Could you check a few things on this model? Use its own coordinates, in mm. Face numbers are marked on the shaded views. A direction names the side the tool comes from. Coordinates: 2 decimals unless noted, no trailing zeros. Loops run counter-clockwise (first coordinate to the right, second up) from the corner with the lowest first, then second, coordinate; pieces in that order, holes last.
Autodesk Inventor part; units mm, degrees
ref_plane "YZ Plane" through (0, 0, 0) normal (1, 0, 0) x (0, 1, 0)
ref_plane "XZ Plane" through (0, 0, 0) normal (0, 1, 0) x (-1, 0, 0)
ref_plane "XY Plane" through (0, 0, 0) normal (0, 0, 1) x (1, 0, 0)
sketch "Skizze1" plane through (0, 0, 0) normal (0, 0, 1) x (1, 0, 0)
  line L0 (0, 0) -> (6.75, 0)
  line L1 (6.75, 0) -> (6.75, 4.9)
  line L2 (6.75, 4.9) -> (3.75, 4.9)
  line L3 (3.75, 4.9) -> (3.75, 10.2)
  line L4 (3.75, 10.2) -> (18.25, 10.2)
  line L5 (18.25, 10.2) -> (18.25, 4.9)
  line L6 (18.25, 4.9) -> (15.25, 4.9)
  line L7 (15.25, 4.9) -> (15.25, 0)
  line L8 (15.25, 0) -> (22, 0)
  line L9 (22, 0) -> (22, 80.2)
  line L10 (0, 0) -> (0, 65.0995)
  line L11 (22, 80.2) -> (22, 98.8308) construction
  line L12 (22, 80.2) -> (17.076, 79.3318)
  line L13 (17.076, 79.3318) -> (15.8604, 86.2254)
  arc A0 (22, 87.0995) -> (15.8604, 86.2254) centre (22, 65.0995) ccw construction
  arc A1 (15.8604, 86.2254) -> (0, 65.0995) centre (22, 65.0995) ccw
  dimension "d0" = 14.5
  dimension "d1" = 5.3
  dimension "d2" = 4.9
  dimension "d3" = 22
  dimension "d4" = 8.5
  dimension "d5" = 5
  dimension "d6" = 7
  dimension "d21" = 70
  dimension "d22" = 80
extrude "Extrusion1" add sketch "Skizze1" along normal blind 22
sketch "Skizze2" plane through (22, 0, 0) normal (1, 0, 0) x (0, 0, -1)
  circle A0 centre (-11, 7.5) radius 2
  line L0 (0, 0) -> (-22, 0)
  line L1 (0, 0) -> (0, 80.2)
  point P0 (0, 65.2)
  dimension "d10" = 4
  dimension "d11" = 7.5
  dimension "d12" = 11
extrude "Extrusion2" cut sketch "Skizze2" against normal blind 22
chamfer "Fasen1" distance 1 angle 45 18 edges at (3.75, 7.55, 22) (11, 10.2, 22) (18.25, 7.55, 22) (16.75, 4.9, 22) (5.25, 4.9, 22) (6.75, 2.45, 22) (15.25, 2.45, 22) (18.25, 7.55, 0) (15.25, 2.45, 0) (16.75, 4.9, 0) (11, 10.2, 0) (3.75, 7.55, 0) (5.25, 4.9, 0) (6.75, 2.45, 0) (6.75, 4.9, 11) (15.25, 4.9, 11) (6.75, 0, 11) (15.25, 0, 11)
properties part number "Gripper_V2_10deg"
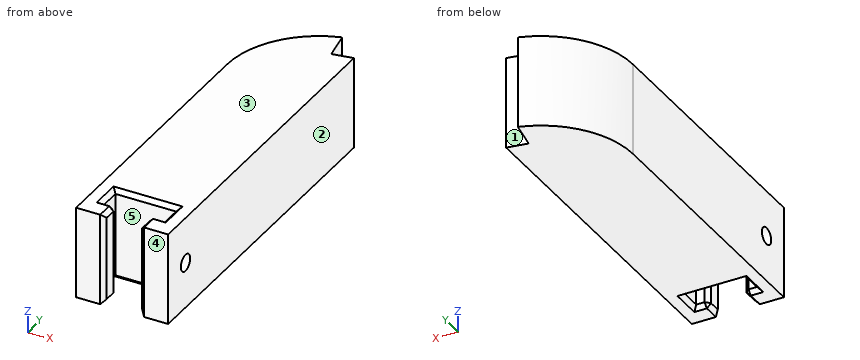
(1) For pin 1 (1 mm diameter, centred on x = 11.5, y = 53, fed in from -Z); pin 2 (4 mm diameter, centred on y = 74.5, z = 3, fed in from -X); pin 3 (0.6 mm diameter, centred on x = 5, z = 9, fed in from +Y), each with a flat end and sliding along its axis, tell me the tip position at first contact or that it passes through.
Answers:
pin 1: stops at z = 0
pin 2: stops at x = 1.28
pin 3: stops at y = 79.42
(2) We'd pull the mould along Y, two halves only. Please class the marked faces 3, 4 and 5: +Y half, -Y half, draft (parallel to the pull), parting line (faces both ways), or undercut.
Answers:
face 3: draft
face 4: -Y half
face 5: undercut
(3) Imagine slicing it at A-A, the plane z = 11. Write out the boundary of the cut face in (x, y).
Answers:
outline: (0, 0) - (5.75, 0) - (6.75, 1) - (6.75, 3.9) - (5.75, 4.9) - (3.75, 4.9) - (3.75, 5.5) - (0, 5.5) - close; (0, 9.5) - (3.75, 9.5) - (3.75, 10.2) - (18.25, 10.2) - (18.25, 9.5) - (22, 9.5) - (22, 80.2) - (17.08, 79.33) - (15.86, 86.23) arc R22 ccw to (0, 65.1) - close; (15.25, 1) - (16.25, 0) - (22, 0) - (22, 5.5) - (18.25, 5.5) - (18.25, 4.9) - (16.25, 4.9) - (15.25, 3.9) - close
(4) Which directions (+Z, -Z, +X, -X, +Y, -Y) give clear straight access to the entire face, cutting with the end or side of a thin tool? Please do the marked faces 1 and 2.
Answers:
face 1: +Z, -Z, +Y
face 2: +Z, -Z, +X, +Y, -Y
(5) Imagine slicing it at C-C, the plane x = 14.5. Write out the boundary of the cut face in (y, z), and give its area (3 significant figures).
Answers:
outline: (10.2, 1) - (11.2, 0) - (85.78, 0) - (85.78, 22) - (11.2, 22) - (10.2, 21) - close
area: 1,660 mm2
(6) I need wall thicknesses on probe 1 along X at (y, z) = (6, 4); probe 2 along Y at (x, z) = (2.75, 11.5); probe 3 along Y at (x, z) = (20.8, 11). Which ranges of each line are inside material? Lowest first, please.
Answers:
probe 1: x = 0 to 3.75, 18.25 to 22
probe 2: y = 0 to 5.56, 9.44 to 75.75
probe 3: y = 0 to 5.5, 9.5 to 79.99
(7) Imagine slicing it at D-D, the plane y = 70.5. Write out the boundary of the cut face in (x, z).
Answers:
outline: (0.67, 0) - (22, 0) - (22, 22) - (0.67, 22) - close
(8) Imagine slicing it at B-B, the plane y = 7.5. Write out the boundary of the cut face in (x, z), and give its area (3 significant figures).
Answers:
outline: (0, 0) - (2.75, 0) - (3.75, 1) - (3.75, 9) - (0, 9) - close; (0, 13) - (3.75, 13) - (3.75, 21) - (2.75, 22) - (0, 22) - close; (18.25, 1) - (19.25, 0) - (22, 0) - (22, 9) - (18.25, 9) - close; (18.25, 13) - (22, 13) - (22, 22) - (19.25, 22) - (18.25, 21) - close
area: 133 mm2
